from build123d import *

# Parameters (mm, degrees)
F0_R     = 130
F1_DEPTH = 5
F2_R     = 2.75
F2_R_2   = 4.25
F3_DEPTH = 5.001


with BuildPart() as f1:
    # F0 (on Top) → F1 (new body)
    with BuildSketch(Plane.XY):
        Circle(F0_R)
    extrude(amount=F1_DEPTH)

    # F2 (on face) → F3 (cut, through all)
    with BuildSketch(Plane.XY.offset(5)):
        Circle(F2_R)
        with Locations((0, 115)):
            Circle(F2_R_2)
        with Locations((-99.592921, -57.5)):
            Circle(F2_R_2)
        with Locations((99.592921, -57.5)):
            Circle(F2_R_2)
    extrude(amount=-F3_DEPTH, mode=Mode.SUBTRACT)


solid = f1.part
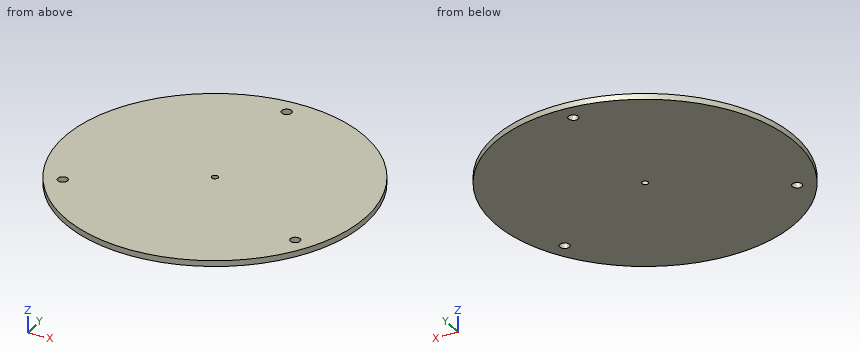
CAD build for the part. Positions are in the model's coordinates, mm. Give positions to 0.01 mm unless a question says otherwise; leave off trailing zeros. Write each loop counter-clockwise with the first axis right and the second up, starting at its lowest first coordinate (ties: lowest second). Pieces come first, ordered by that corner, then holes. Notation, with made-up numbers: (-38.75, 59.5) - (0.25, 59.5) arc R25 ccw to (0.25, 88.5) - close; hole circle Ø4 at (-2, 8.5). An arc over 180 degrees is marked (long way). Answer as CSV lines item,"result".
Q1. Band-saw the part on C-C (y = -32). Give the cut face in (x, z), and give its area (3 significant figures).
Result set:
outline,"(-126, 0) - (126, 0) - (126, 5) - (-126, 5) - close"
area,"1,260 mm²"
Q2. Band-saw the part on A-A (z = 2). Give the cut face in (x, y), and give its area (3 significant figures).
Result set:
outline,"circle Ø260 at (0, 0); hole circle Ø8.5 at (-99.59, -57.5); hole circle Ø8.5 at (0, 115); hole circle Ø5.5 at (0, 0); hole circle Ø8.5 at (99.59, -57.5)"
area,"52,900 mm²"
Q3. Band-saw the part on D-D (x = -110.5). Give the cut face in (y, z).
Result set:
outline,"(-68.48, 0) - (68.48, 0) - (68.48, 5) - (-68.48, 5) - close"
Q4. Flat gauge pin, fed straight in: pin 1 Ø3 at (y, z) = (-59, 2.5) entering from -X. Where does the tip first touch, or does it go through?
Result set:
pin 1,"x = -116.59"
Q5. Drill centre lines: line 1 (Y direction, x = 0, z = 1.3); line 2 (Y direction, x = 14, z = 0.3); line 3 (X direction, y = 98, z = 1.4). Where is each one in solid material? Low to high. Write a range as from..to.
Result set:
line 1,"-130..-2.75, 2.75..110.75, 119.25..130"
line 2,"-129.24..129.24"
line 3,"-85.42..85.42"
Q6. Band-saw the part on B-B (y = 115). Give the cut face in (x, z).
Result set:
outline,"(-60.62, 0) - (-4.25, 0) - (-4.25, 5) - (-60.62, 5) - close; (4.25, 0) - (60.62, 0) - (60.62, 5) - (4.25, 5) - close"
